Autodesk Inventor part; units mm, degrees
ref_plane "YZ Plane" through (0, 0, 0) normal (1, 0, 0) x (0, 1, 0)
ref_plane "XZ Plane" through (0, 0, 0) normal (0, 1, 0) x (-1, 0, 0)
ref_plane "XY Plane" through (0, 0, 0) normal (0, 0, 1) x (1, 0, 0)
sketch "スケッチ1" plane through (0, 0, 0) normal (0, 0, 1) x (1, 0, 0)
  circle A0 centre (0, 0) radius 30
  circle A1 centre (0, 0) radius 25
  dimension "d0" = 60
  dimension "d1" = 5
extrude "押し出し1" add sketch "スケッチ1" along normal mid plane 8
sketch "スケッチ2" plane through (0, 0, 0) normal (0, 0, 1) x (1, 0, 0)
  circle A0 centre (0, 0) radius 9.35
  line L0 (-1.5, 26) -> (-2.5, 0)
  line L1 (-2.5, 0) -> (2.5, 0)
  line L2 (2.5, 0) -> (1.5, 26)
  line L3 (1.5, 26) -> (-1.5, 26)
  point P0 (0, 26)
  point P1 (-2.15, 9.0994)
  point P2 (2.15, 9.0994)
  dimension "d4" = 18.7
  dimension "d5" = 5
  dimension "d6" = 3
  dimension "d7" = 26
extrude "押し出し2" add sketch "スケッチ2" along normal mid plane 5
pattern_circular "円形状パターン1" count 5 over 360 about axis through (0, 0, -10) along (0, 0, 1) of "押し出し2"
sketch "スケッチ3" plane through (0, 0, -2.5) normal (0, 0, -1) x (-1, 0, 0)
  circle A0 centre (0, 0) radius 3
  dimension "d13" = 6
extrude "押し出し3" add sketch "スケッチ3" along normal blind 3
sketch "スケッチ4" plane through (0, 0, -5.5) normal (0, 0, -1) x (-1, 0, 0)
  circle A0 centre (0, 0) radius 2.43
  dimension "d16" = 4.86
extrude "押し出し4" cut sketch "スケッチ4" against normal blind 3
properties part number "FS90R-W"
The listing builds one solid part. Answer for the finished solid, in the listing's coordinates (mm). A direction names the side the tool comes from. Give positions to 0.01 mm unless a question says otherwise; leave off trailing zeros. Write each loop counter-clockwise with the first axis right and the second up, starting at its lowest first coordinate (ties: lowest second). Pieces come first, ordered by that corner, then holes. Notation, with made-up numbers: (75, 8) -> (85, 8) arc R12 cw to (85, 24) -> close; hole circle Ø9 at (22, -36). An arc over 180 degrees is marked (long way). Use a Markdown table: item, result.
(1) Section D-D, the plane x = -15 is taken. Determine the outline of the cut face in (y, z).
Return value:
| item | result |
|---|---|
| outline | (-25.98, -4) -> (-20, -4) -> (-20, -2.5) -> (-17.92, -2.5) -> (-17.92, 2.5) -> (-20, 2.5) -> (-20, 4) -> (-25.98, 4) -> close; (2.86, -2.5) -> (6.84, -2.5) -> (6.84, 2.5) -> (2.86, 2.5) -> close; (20, -4) -> (25.98, -4) -> (25.98, 4) -> (20, 4) -> close |
(2) Section B-B, the plane y = 0 is taken. Determine the outline of the cut face in (x, z), then the cut area to 3 significant figures.
Return value:
| item | result |
|---|---|
| outline | (-30, -4) -> (-25, -4) -> (-25, 4) -> (-30, 4) -> close; (-9.35, -2.5) -> (-3, -2.5) -> (-3, -5.5) -> (-2.43, -5.5) -> (-2.43, -2.5) -> (2.43, -2.5) -> (2.43, -5.5) -> (3, -5.5) -> (3, -2.5) -> (9.35, -2.5) -> (9.35, 2.5) -> (-9.35, 2.5) -> close; (25, -4) -> (30, -4) -> (30, 4) -> (25, 4) -> close |
| area | 177 mm2 |
(3) Section C-C, the plane z = -1.5 is taken. Determine the outline of the cut face in (x, y), then the cut area to 3 significant figures.
Return value:
| item | result |
|---|---|
| outline | circle Ø60 at (0, 0); hole (-24.21, 6.25) arc R25 ccw to (-15.91, -19.28) -> (-7.09, -6.1) arc R9.35 cw to (-9.32, 0.77) -> close; hole (-23.26, 9.18) -> (-7.99, 4.86) arc R9.35 cw to (-2.15, 9.1) -> (-1.54, 24.95) arc R25 ccw to start; hole (-13.42, -21.09) arc R25 ccw to (13.42, -21.09) -> (3.61, -8.63) arc R9.35 cw to (-3.61, -8.63) -> close; hole (1.54, 24.95) -> (2.15, 9.1) arc R9.35 cw to (7.99, 4.86) -> (23.26, 9.18) arc R25 ccw to start; hole (7.09, -6.1) -> (15.91, -19.28) arc R25 ccw to (24.21, 6.25) -> (9.32, 0.77) arc R9.35 cw to start |
| area | 1,430 mm2 |
(4) For faces 1 (the flat face through (15.729, 7.046, -0.035)), 2 (the cylindrical face through (1.928, -1.479, -4.021)), determine the directions among +Z, -Z, +X, -X, +Y, -Y from which every point of the face is accessible in a straight line to the end or side of a thin tool.
Return value:
| item | result |
|---|---|
| face 1 | +Z, -Z |
| face 2 | -Z |
(5) Find the intervals of material crossed by probe 1 along Y at (x, z) = (0, -3.45); probe 2 along Y at (x, z) = (0, -0.5); probe 3 along X at (y, z) = (-3, -0.25), in increasing order. Write a range as from..to.
Return value:
| item | result |
|---|---|
| probe 1 | -30..-25, -3..-2.43, 2.43..3, 25..30 |
| probe 2 | -30..-25, -9.35..30 |
| probe 3 | -29.85..-24.82, -8.86..8.86, 24.82..29.85 |
(6) Flat-ended cylindrical pins translate along their axes: P1, Ø1.5, axis at y = 16.5, z = 0, coming from the +X side; P2, Ø1.5, axis at x = -0.5, y = 1, coming from the -Z side; P3, Ø14, axis at x = -9.5, y = 5, coming from the +Z side; P4, Ø10, axis at x = 17.5, y = -2.5, coming from the +Z side. Find the tip coordinate at first contact, or state that the pin passes through.
Return value:
| item | result |
|---|---|
| P1 | x = 25.53 |
| P2 | z = -2.5 |
| P3 | z = 2.5 |
| P4 | through |
(7) Section A-A, the plane x = 0 is taken. Determine the outline of the cut face in (y, z).
Return value:
| item | result |
|---|---|
| outline | (-30, -4) -> (-25, -4) -> (-25, 4) -> (-30, 4) -> close; (-9.35, -2.5) -> (-3, -2.5) -> (-3, -5.5) -> (-2.43, -5.5) -> (-2.43, -2.5) -> (2.43, -2.5) -> (2.43, -5.5) -> (3, -5.5) -> (3, -2.5) -> (25, -2.5) -> (25, -4) -> (30, -4) -> (30, 4) -> (25, 4) -> (25, 2.5) -> (-9.35, 2.5) -> close |
(8) Determine the mould class of faces 3 (the flat face through (-7, 25, 4)), 4 (the cylindrical face through (-8.876, -2.939, -0.035)), 5 (the cylindrical face through (-29.97, -1.32, -0.06)) for opening direction X: released by +X, released by -X, zero draft, split by the parting line, or undercut.
Return value:
| item | result |
|---|---|
| face 3 | zero draft |
| face 4 | undercut |
| face 5 | split by the parting line |
